Model file for the job. Use its own axes, mm. A direction names the side the tool comes from. Round coordinates to 2 decimals unless told otherwise and drop trailing zeros. Loops run counter-clockwise (first coordinate to the right, second up) from the corner with the lowest first, then second, coordinate; pieces in that order, holes last. Notation, with made-up numbers: (46, 16.25) -> (99, 16.25) arc R22 cw to (99, 52.25) -> close; hole circle Ø6 at (-2, -39.75). An arc over 180 degrees is marked (long way). Use a Markdown table: item, result.
from build123d import *

# Parameters (mm, degrees)
SKETCH1_W           = 152.4
SKETCH1_H           = 114.3
BOSS_EXTRUDE1_DEPTH = 3.18
SKETCH2_OUTSIDE_W   = 192.506
SKETCH2_OUTSIDE_H   = 154.406
CUT_EXTRUDE2_DEPTH  = 3.18


with BuildPart() as part:
    # Sketch1 → Boss-Extrude1 (new body)
    with BuildSketch(Plane.XY):
        Rectangle(SKETCH1_W, SKETCH1_H)
    extrude(amount=BOSS_EXTRUDE1_DEPTH)

    # Sketch2 outside → Cut-Extrude2 (cut)
    with BuildSketch(Plane.XY.offset(3.18)):
        Rectangle(SKETCH2_OUTSIDE_W, SKETCH2_OUTSIDE_H)
        with BuildLine():
            Line((48.053666352, -28.069013415), (48.053666352, -48.069013415))
            Line((48.053666352, -48.069013415), (51.553666352, -48.069013415))
            Line((51.553666352, -48.069013415), (51.553666352, -51.069013415))
            Line((51.553666352, -51.069013415), (40.553666352, -51.069013415))
            Line((40.553666352, -51.069013415), (40.553666352, -48.069013415))
            Line((40.553666352, -48.069013415), (44.053666352, -48.069013415))
            Line((44.053666352, -48.069013415), (44.053666352, -34.069013415))
            Line((44.053666352, -34.069013415), (39.278768341, -34.069013415))
            Line((39.278768341, -34.069013415), (39.278768341, -31.069013415))
            ThreePointArc((39.278768341, -31.069013415), (42.983469512, -30.28546377), (46.053666352, -28.069013415))
            Line((46.053666352, -28.069013415), (48.053666352, -28.069013415))
        make_face(mode=Mode.SUBTRACT)
    extrude(amount=-CUT_EXTRUDE2_DEPTH, mode=Mode.SUBTRACT)


solid = part.part
Q1. Band-saw the part on A-A, the plane z = 2.35. Give the cut face in (x, y).
Results list:
| item | result |
|---|---|
| outline | (39.28, -34.07) -> (44.05, -34.07) -> (44.05, -48.07) -> (40.55, -48.07) -> (40.55, -51.07) -> (51.55, -51.07) -> (51.55, -48.07) -> (48.05, -48.07) -> (48.05, -28.07) -> (46.05, -28.07) arc R9.15 cw to (39.28, -31.07) -> close |
Q2. Band-saw the part on B-B, the plane x = 41.5. Give the cut face in (y, z).
Results list:
| item | result |
|---|---|
| outline | (-51.07, 0) -> (-48.07, 0) -> (-48.07, 3.18) -> (-51.07, 3.18) -> close; (-34.07, 0) -> (-30.8, 0) -> (-30.8, 3.18) -> (-34.07, 3.18) -> close |
Q3. Band-saw the part on D-D, the plane x = 49.75. Give the cut face in (y, z).
Results list:
| item | result |
|---|---|
| outline | (-51.07, 0) -> (-48.07, 0) -> (-48.07, 3.18) -> (-51.07, 3.18) -> close |
Q4. Pull direction Y, two halves, no side cores. Call faces 4 (the face through (47, -28.069, 2)), 5 (the face through (42, -48.069, 2)), 6 (the face through (46, -51.069, 2)), 7 (the face through (40.554, -50, 2)): released by +Y, released by -Y, zero draft, split by the parting line, or undercut.
Results list:
| item | result |
|---|---|
| face 4 | released by +Y |
| face 5 | undercut |
| face 6 | released by -Y |
| face 7 | zero draft |
Q5. Band-saw the part on C-C, the plane y = -36.5. Give the cut face in (x, z), plus the area to 3 significant figures.
Results list:
| item | result |
|---|---|
| outline | (44.05, 0) -> (48.05, 0) -> (48.05, 3.18) -> (44.05, 3.18) -> close |
| area | 12.7 mm² |
Q6. Drill centre lines: L1, parallel to Y at x = 50, z = 2.8; L2, parallel to Y at x = 42, z = 2.4 (3 decimals); L3, parallel to X at y = -42.5, z = 0.65. Where is each one in solid material? Low to high. Write a range as from..to.
Results list:
| item | result |
|---|---|
| L1 | y = -51.07..-48.07 |
| L2 | y = -51.069..-48.069, -34.069..-30.655 |
| L3 | x = 44.05..48.05 |
Q7. Tool access for faces 1 (the face through (46, -40, 0)), 2 (the face through (44.054, -41, 2)), 3 (the face through (50, -48.069, 2)): list every direction of +Z, -Z, +X, -X, +Y, -Y with a clear straight run to the whole face (end or side of a thin tool).
Results list:
| item | result |
|---|---|
| face 1 | -Z, +X, -X, +Y, -Y |
| face 2 | +Z, -Z, -X |
| face 3 | +Z, -Z, +X, +Y |
Q8. Flat gauge pins, fed straight in: pin 1 (1 mm diameter, centred on x = 50, z = 1, fed in from +Y); pin 2 (1.5 mm diameter, centred on y = -49.5, z = 2.5, fed in from -X); pin 3 (1.6 mm diameter, centred on y = -37.5, z = 1, fed in from +X). Where does each tip first touch, or does it go through?
Results list:
| item | result |
|---|---|
| pin 1 | stops at y = -48.07 |
| pin 2 | stops at x = 40.55 |
| pin 3 | stops at x = 48.05 |
